Input: part model. Units: mm. Frame: model coordinates. Face numbers are marked on the shaded views. Give positions to 0.01 mm unless a question says otherwise; leave off trailing zeros. Loops run counter-clockwise (first coordinate to the right, second up) from the corner with the lowest first, then second, coordinate; pieces in that order, holes last. Notation, with made-up numbers: (34.5, 78) - (65.5, 78) arc R26 ccw to (65.5, 103) - close; hole circle Ø9 at (33, 21.5). An arc over 180 degrees is marked (long way). Answer as a JSON object with one key per item and string values. Group by question number.
(1) Material intervals for L1, parallel to X at y = 3.5, z = 24; L2, parallel to X at y = 9.5, z = 43; L3, parallel to Y at x = 16, z = 44, sorted ascending.
(2) Mould query, pull axis X, two halves, no side actions, for the marked faces 1, 2 and 3. Classes: +X half, -X half, draft (parallel to the pull), parting line (faces both ways), or undercut.
(3) Section query D-D (y = 5.25). Return loops of the section in (x, z).
(4) Section query A-A (y = 10). Return loops of the section in (x, z).
(5) Section query C-C (x = 15.88). Return loops of the section in (y, z).
(6) Pin query (flat end, axial travel): P1, Ø5, axis at x = 15.5, z = 38.5, coming from the -Y side. Return the tip coordinate at first contact, or that it passes through.
```python
from build123d import *

# Parameters (mm, degrees)
CROQUIS2_W              = 76.2
CROQUIS2_H              = 50.8
CROQUIS2_R              = 9.525
SALIENTE_EXTRUIR1_DEPTH = 50.8
CROQUIS3_W              = 76.2
CROQUIS3_H              = 25.4
CORTAR_EXTRUIR1_DEPTH   = 50.8
CORTAR_EXTRUIR2_DEPTH   = 50.8


with BuildPart() as part:
    # Croquis2 → Saliente-Extruir1 (new body)
    with BuildSketch(Plane.XY):
        with Locations((39.6925, 0)):
            Rectangle(CROQUIS2_W, CROQUIS2_H)
        with Locations((15.88, 0)):
            Circle(CROQUIS2_R, mode=Mode.SUBTRACT)
        with Locations((63.505, 0)):
            Circle(CROQUIS2_R, mode=Mode.SUBTRACT)
    extrude(amount=SALIENTE_EXTRUIR1_DEPTH)

    # Croquis3 → Cortar-Extruir1 (cut)
    with BuildSketch(Plane.XY.offset(50.8)):
        with Locations((39.6925, -12.7)):
            Rectangle(CROQUIS3_W, CROQUIS3_H)
    extrude(amount=-CORTAR_EXTRUIR1_DEPTH, mode=Mode.SUBTRACT)

    # Croquis4 → Cortar-Extruir2 (cut)
    with BuildSketch(Plane.XY.offset(50.8)):
        with BuildLine():
            Line((6.355, 0), (6.355, 3.175))
            ThreePointArc((6.355, 3.175), (15.88, 12.7), (25.405, 3.175))
            Line((25.405, 3.175), (25.405, 0))
            Line((25.405, 0), (6.355, 0))
        make_face()
        with BuildLine():
            Line((73.03, 0), (53.98, 0))
            Line((53.98, 0), (53.98, 3.175))
            ThreePointArc((53.98, 3.175), (63.505, 12.7), (73.03, 3.175))
            Line((73.03, 3.175), (73.03, 0))
        make_face()
    extrude(amount=-CORTAR_EXTRUIR2_DEPTH, mode=Mode.SUBTRACT)


solid = part.part
```
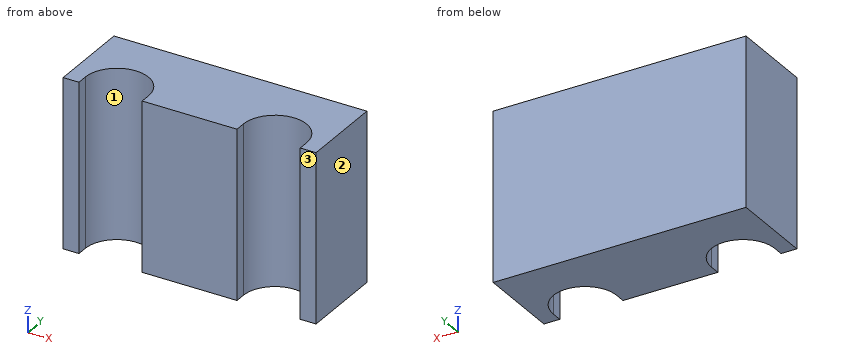
Recorded:
{
 "1": {"L1": "x = 1.59 to 6.36, 25.4 to 53.99, 73.02 to 77.79", "L2": "x = 1.59 to 8.76, 23 to 56.38, 70.63 to 77.79", "L3": "y = 12.7 to 25.4"},
 "2": {"face 1": "undercut", "face 2": "+X half", "face 3": "draft"},
 "3": {"outline": "(1.59, 0) - (6.58, 0) - (6.58, 50.8) - (1.59, 50.8) - close; (25.18, 0) - (54.21, 0) - (54.21, 50.8) - (25.18, 50.8) - close; (72.8, 0) - (77.79, 0) - (77.79, 50.8) - (72.8, 50.8) - close"},
 "4": {"outline": "(1.59, 0) - (9.24, 0) - (9.24, 50.8) - (1.59, 50.8) - close; (22.52, 0) - (56.86, 0) - (56.86, 50.8) - (22.52, 50.8) - close; (70.15, 0) - (77.79, 0) - (77.79, 50.8) - (70.15, 50.8) - close"},
 "5": {"outline": "(12.7, 0) - (25.4, 0) - (25.4, 50.8) - (12.7, 50.8) - close"},
 "6": {"P1": "stops at y = 12.25"}
}
